Geometry: final body of the model. Coordinates: model frame, mm. A direction names the side the tool comes from. Give positions to 0.01 mm unless a question says otherwise; leave off trailing zeros. Write each loop counter-clockwise with the first axis right and the second up, starting at its lowest first coordinate (ties: lowest second). Pieces come first, ordered by that corner, then holes.
Q1. Cut plane C-C on x = 10.5. Return the cut outline in (y, z) (3 decimals).
Q2. Cut plane A-A on z = 40. Return the cut outline in (x, y), plus the area to 3 significant figures.
Q3. Pin query (flat end, axial travel): pin 1 (12 mm diameter, centred on x = -76.5, z = 23, fed in from -Y); pin 2 (12 mm diameter, centred on x = -31.5, z = 16, fed in from +Y). Return the tip coordinate at first contact, or that it passes through.
Q4. Draft query along Y for faces 4 (the face through (-36, -39.324, 44)), 5 (the face through (65.091, 88, 42)), 6 (the face through (55, -87.214, 42)). Return one class per face: pulls with the +Y half, pulls with the -Y half, needs draft (parallel to the pull), parting line crosses it, or undercut.
Q5. Cut plane B-B on y = -65.5. Return the cut outline in (x, z) (3 decimals), plus the area to 3 significant figures.
Q6. Line query: L1, parallel to X at y = -66, z = 13; L2, parallel to X at y = 20.5, z = 25; L3, parallel to Y at x = -111, z = 16.5. Output: solid intervals per line, ascending.
Q7. Cut plane D-D on y = -36.5. Return the cut outline in (x, z) (3 decimals).
Q8. Reachability of faces 1 (the face through (-169.859, 9, 42)), 2 (the face through (-87.309, -65, 42)), 3 (the face through (68.266, 84, 44)) from +Z, -Z, +X, -X, +Y, -Y: full face, straight path, thin tool, end or side. Return the list, or none.
```python
from build123d import *

# Parameters (mm, degrees)
F1_DEPTH = 3.175
F3_DEPTH = 88.9
F4_W     = 50.8
F4_H     = 38.1
F5_DEPTH = 95.25


with BuildPart() as f1:
    # F0 (on Top) → F1 (new body)
    with BuildSketch(Plane.XY):
        Polygon((-138.109116, 103.285787), (-169.859116, 103.285787), (-169.859116, -87.214213), (-87.309116, -87.214213), (-87.309116, -42.498762), (14.290884, -42.498762), (14.290884, -87.214213), (96.840884, -87.214213), (96.840884, 103.285787), (65.090884, 103.285787), (65.090884, 71.801238), (-138.109116, 71.801238), align=None)
    extrude(amount=-F1_DEPTH)

    # F2 (on face) → F3 (join)
    with BuildSketch(Plane.XY):
        Polygon((-138.109116, 103.285787), (-169.859116, 103.285787), (-169.859116, -87.214213), (-87.309116, -87.214213), (-87.309116, -42.498762), (14.290884, -42.498762), (14.290884, -87.214213), (96.840884, -87.214213), (96.840884, 103.285787), (65.090884, 103.285787), (65.090884, 71.801238), (-138.109116, 71.801238), align=None)
        Polygon((-166.684116, -84.039213), (-166.684116, 100.110787), (-141.284116, 100.110787), (-141.284116, 68.626238), (68.265884, 68.626238), (68.265884, 100.110787), (93.665884, 100.110787), (93.665884, -84.039213), (40.343958, -84.039213), (17.465884, -84.039213), (17.465884, -39.323762), (-90.484116, -39.323762), (-90.484116, -84.039213), (-116.960541, -84.039213), align=None, mode=Mode.SUBTRACT)
    extrude(amount=F3_DEPTH)

    # F4 (on face) → F5 (join)
    with BuildSketch(Plane.XY):
        with Locations((-36.509116, 14.651238)):
            Rectangle(F4_W, F4_H)
    extrude(amount=F5_DEPTH)


solid = f1.part
```
Data:
1. outline: (-42.499, -3.175) - (71.801, -3.175) - (71.801, 88.9) - (68.626, 88.9) - (68.626, 0) - (-39.324, 0) - (-39.324, 88.9) - (-42.499, 88.9) - close
2. outline: (-169.86, -87.21) - (-87.31, -87.21) - (-87.31, -42.5) - (14.29, -42.5) - (14.29, -87.21) - (96.84, -87.21) - (96.84, 103.29) - (65.09, 103.29) - (65.09, 71.8) - (-138.11, 71.8) - (-138.11, 103.29) - (-169.86, 103.29) - close; (-61.91, -4.4) - (-11.11, -4.4) - (-11.11, 33.7) - (-61.91, 33.7) - close; hole (-166.68, -84.04) - (-90.48, -84.04) - (-90.48, -39.32) - (17.47, -39.32) - (17.47, -84.04) - (93.67, -84.04) - (93.67, 100.11) - (68.27, 100.11) - (68.27, 68.63) - (-141.28, 68.63) - (-141.28, 100.11) - (-166.68, 100.11) - close
2. area: 5,280 mm2
3. pin 1: stops at y = -42.5
3. pin 2: stops at y = 71.8
4. face 4: undercut
4. face 5: needs draft
4. face 6: pulls with the -Y half
5. outline: (-169.859, -3.175) - (-87.309, -3.175) - (-87.309, 88.9) - (-90.484, 88.9) - (-90.484, 0) - (-166.684, 0) - (-166.684, 88.9) - (-169.859, 88.9) - close; (14.291, -3.175) - (96.841, -3.175) - (96.841, 88.9) - (93.666, 88.9) - (93.666, 0) - (17.466, 0) - (17.466, 88.9) - (14.291, 88.9) - close
5. area: 1,650 mm2
6. L1: x = -169.86 to -166.68, -90.48 to -87.31, 14.29 to 17.47, 93.67 to 96.84
6. L2: x = -169.86 to -166.68, -61.91 to -11.11, 93.67 to 96.84
6. L3: y = -87.21 to -84.04, 68.63 to 71.8
7. outline: (-169.859, -3.175) - (96.841, -3.175) - (96.841, 88.9) - (93.666, 88.9) - (93.666, 0) - (-166.684, 0) - (-166.684, 88.9) - (-169.859, 88.9) - close
8. face 1: +Z, -Z, -X, +Y, -Y
8. face 2: +Z, -Z, -Y
8. face 3: +Z
